Input: dimensioned drawing with shaded views. Units: mm. Origin: part minimum x, y, z. Round coordinates to 2 decimals unless told otherwise and drop trailing zeros. Write each loop counter-clockwise with the first axis right and the second up, starting at its lowest first coordinate (ties: lowest second). Pieces come first, ordered by that corner, then holes. Notation, with made-up numbers: (-38, 8) - (-9, 8) arc R17 ccw to (-9, 18) - close; hole circle Ø2 at (88, 49.25). An arc over 180 degrees is marked (long way). Write item = value, one per line. Start each with the question number.
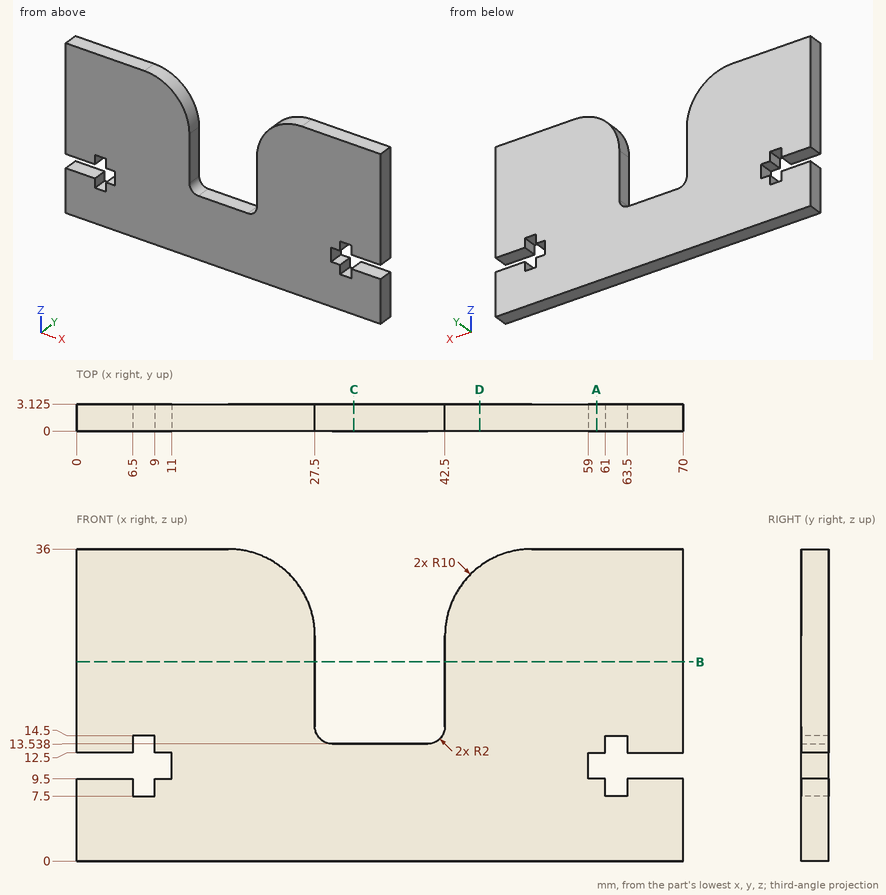
(1) Section A-A (x = 60). Return the cut outline in (y, z) (1 decimal).
(2) Section D-D (x = 46.5). Return the cut outline in (y, z) (1 decimal).
(3) Section C-C (x = 32). Return the cut outline in (y, z) (1 decimal), plus the area to 3 significant figures.
(4) Contact query for flat-ended pins moving along their axis: P1, Ø0.6, axis at y = 1, z = 9, coming from the -X side; P2, Ø1.5, axis at y = 1, z = 11, coming from the +X side. Output: stop coordinate, or through.
(5) Ray query, L1, parallel to X at y = 2.3, z = 24; L2, parallel to Z at x = 8, y = 0.7; L3, parallel to Z at x = 64.5, y = 1.2. Return the intervals inside material, ascending. Write a range as from..to.
(6) Section B-B (z = 23). Return the cut outline in (x, y) (1 decimal), plus the area to 3 significant figures.
Solution:
q1.outline = (0, 0) - (3.1, 0) - (3.1, 9.5) - (0, 9.5) - close; (0, 12.5) - (3.1, 12.5) - (3.1, 36) - (0, 36) - close
q2.outline = (0, 0) - (3.1, 0) - (3.1, 34) - (0, 34) - close
q3.outline = (0, 0) - (3.1, 0) - (3.1, 13.5) - (0, 13.5) - close
q3.area = 42.3 mm^2
q4.P1 = 0
q4.P2 = 59
q5.L1 = 0..27.5, 42.5..70
q5.L2 = 0..7.5, 14.5..36
q5.L3 = 0..9.5, 12.5..36
q6.outline = (0, 0) - (27.5, 0) - (27.5, 3.1) - (0, 3.1) - close; (42.5, 0) - (70, 0) - (70, 3.1) - (42.5, 3.1) - close
q6.area = 172 mm^2
